Source: CAD feature listing. Evaluate the final solid. Frame: model axes, mm. A direction names the side the tool comes from. Round coordinates to 2 decimals unless told otherwise and drop trailing zeros. Answer as CSV lines item,"result".
from build123d import *

# Parameters (mm, degrees)
SKETCH2_W           = 30
SKETCH2_H           = 30
BOSS_EXTRUDE1_DEPTH = 50
SKETCH3_W           = 25
SKETCH3_H           = 25
CUT_EXTRUDE1_DEPTH  = 2.5
FILLET1_R           = 5
SKETCH9_W           = 12.5
SKETCH9_H           = 20.172460503
CUT_EXTRUDE2_DEPTH  = 2.5
CIRPATTERN1_COUNT   = 4
FILLET2_R           = 2.5


with BuildPart() as part:
    # Sketch2 → Boss-Extrude1 (new body)
    with BuildSketch(Plane(origin=(0, 0, 0), x_dir=(1, 0, 0), z_dir=(0, 1, 0))):
        Rectangle(SKETCH2_W, SKETCH2_H)
    extrude(amount=BOSS_EXTRUDE1_DEPTH)

    # Sketch3 → Cut-Extrude1 (cut)
    with BuildSketch(Plane(origin=(0, 50, 0), x_dir=(1, 0, 0), z_dir=(0, 1, 0))):
        Rectangle(SKETCH3_W, SKETCH3_H)
    extrude(amount=-CUT_EXTRUDE1_DEPTH, mode=Mode.SUBTRACT)

    # Fillet1
    fillet1_edges = [part.edges().sort_by_distance(p)[0] for p in [
        (15, 25, 15),
        (-15, 25, 15),
        (-15, 25, -15),
        (15, 25, -15),
    ]]
    fillet(fillet1_edges, radius=FILLET1_R)

    # Cut-Loft2: read off the stored shape, not the designer's step
    # Cut-Loft2: loft between two sections, ruled curve by curve
    cut_loft2_from = [
        Edge.make_bspline([(0, 0, -12.5), (-25, 0, -12.5), (-25, 0, 12.5), (0, 0, 12.5), (25, 0, 12.5), (25, 0, -12.5), (0, 0, -12.5)], [0, 0, 0, 0, 0.5, 0.5, 0.5, 1, 1, 1, 1], 3, [1, 0.333333333, 0.333333333, 1, 0.333333333, 0.333333333, 1]),
    ]
    cut_loft2_to = [
        Edge.make_bspline([(0.784484005, 47.5, -2.373728048), (-3.962972092, 47.5, -3.942696057), (-5.531940101, 47.5, 0.804760039), (-0.784484005, 47.5, 2.373728048), (3.962972092, 47.5, 3.942696057), (5.531940101, 47.5, -0.804760039), (0.784484005, 47.5, -2.373728048)], [0, 0, 0, 0, 0.5, 0.5, 0.5, 1, 1, 1, 1], 3, [1, 0.333333333, 0.333333333, 1, 0.333333333, 0.333333333, 1]),
    ]
    cut_loft2 = Solid(Shell([*[Face.make_surface_from_curves(cut_loft2_from[k], cut_loft2_to[k]) for k in range(1)], Face(Wire(cut_loft2_from)), Face(Wire(cut_loft2_to))]))
    add(cut_loft2, mode=Mode.SUBTRACT)

    # Sketch9 → Cut-Extrude2 (cut)
    with BuildSketch(Plane.XY.offset(15)):
        with Locations((0, 39.913769749)):
            Rectangle(SKETCH9_W, SKETCH9_H)
    cut_extrude2 = extrude(amount=-CUT_EXTRUDE2_DEPTH, mode=Mode.SUBTRACT)

    # CirPattern1: Cut-Loft2, Cut-Extrude2 ×4 about axis
    cirpattern1_axis = Axis((0, 0, 0), (0, 1, 0))
    add([cut_loft2.rotate(cirpattern1_axis, i * 360 / CIRPATTERN1_COUNT) for i in range(1, CIRPATTERN1_COUNT)], mode=Mode.SUBTRACT)
    add([cut_extrude2.rotate(cirpattern1_axis, i * 360 / CIRPATTERN1_COUNT) for i in range(1, CIRPATTERN1_COUNT)], mode=Mode.SUBTRACT)

    # Fillet2
    fillet2_edges = [part.edges().sort_by_distance(p)[0] for p in [
        (13.75, 50, 6.25),
        (13.75, 50, -6.25),
        (6.25, 50, -13.75),
        (-6.25, 50, -13.75),
        (-13.75, 50, -6.25),
        (-13.75, 50, 6.25),
        (-6.25, 50, 13.75),
        (6.25, 50, 13.75),
    ]]
    fillet(fillet2_edges, radius=FILLET2_R)


solid = part.part
1. Line query: L1, parallel to Z at x = 4.5, y = 39.5; L2, parallel to Y at x = -7, z = -10.5; L3, parallel to X at y = 13, z = -7. Output: solid intervals per line, ascending. Write a range as [from, to].
Results below:
L1,"[-12.5, 12.5]"
L2,"[0, 47.5]"
L3,"[-15, -6.76], [6.76, 15]"
2. Pin query (flat end, axial travel): pin 1 (0.8 mm diameter, centred on x = 13, z = 1.5, fed in from +Y); pin 2 (8 mm diameter, centred on x = 0.5, y = 34, fed in from -Z); pin 3 (3 mm diameter, centred on x = 14, y = 35, fed in from -Z). Return the tip coordinate at first contact, or that it passes through.
Results below:
pin 1,"y = 29.83"
pin 2,"z = -12.5"
pin 3,"z = -14.33"
3. Mould query, pull axis X, two halves, no side actions, for faces 5 (the cylindrical face through (7.002, 49.287, 13.732)), 6 (the flat face through (-12.5, 39, 0)), 7 (the cylindrical face through (13.732, 49.287, 7.002)), 8 (the flat face through (0, 39, -12.5)). Classes: released by +X, released by -X, zero draft, split by the parting line, or undercut.
Results below:
face 5,"undercut"
face 6,"released by -X"
face 7,"zero draft"
face 8,"undercut"
4. Reachability of faces 1 (the cylindrical face through (-13.732, 49.287, -7.002)), 2 (the flat face through (14, 29.828, 0)), 3 (the flat face through (-6.25, 39, 14)), 4 (the flat face through (12.5, 49, 9)) from +Z, -Z, +X, -X, +Y, -Y: full face, straight path, thin tool, end or side. Return the list, or none.
Results below:
face 1,"+X, -X, +Y"
face 2,"+X, +Y"
face 3,"+Z, +Y"
face 4,"+Y"
